from build123d import *

# Parameters (mm, degrees)
F0_R        = 2.4
F1_DEPTH    = 7.88
F2_T1_DEPTH = 26.405


# Not quite as in the source:
# - a fillet or chamfer that OpenCascade refuses, or shapes differently, is made with other operations: its cross-section is extruded or revolved along the edge and cut away or added


with BuildPart() as f1:
    # F0 (on Top) → F1 (new body)
    with BuildSketch(Plane.XY):
        Polygon((-48.3995083171, -5.7841986276), (-31.3221290569, -5.7841986276), (-9.0295083171, -5.7841986276), (-9.0295083171, 1.2940158032), (-41.0095083171, 1.2940158032), (-41.0095083171, 17.5958013724), (-48.3995083171, 17.5958013724), align=None)
        with Locations((-44.7195083171, -2.0891986276)):
            Circle(F0_R, mode=Mode.SUBTRACT)
        with Locations((-36.7195083171, -2.0891986276)):
            Circle(F0_R, mode=Mode.SUBTRACT)
        with BuildLine():
            ThreePointArc((-28.7195083171, -4.4891986276), (-31.1195083171, -2.0891986276), (-28.7195083171, 0.3108013724))
            ThreePointArc((-28.7195083171, 0.3108013724), (-26.3195083171, -2.0891986276), (-28.7195083171, -4.4891986276))
        make_face(mode=Mode.SUBTRACT)
        with BuildLine():
            ThreePointArc((-20.7195083171, -4.4891986276), (-23.1195083171, -2.0891986276), (-20.7195083171, 0.3108013724))
            ThreePointArc((-20.7195083171, 0.3108013724), (-18.3195083171, -2.0891986276), (-20.7195083171, -4.4891986276))
        make_face(mode=Mode.SUBTRACT)
        with BuildLine():
            ThreePointArc((-12.7195083171, -4.4891986276), (-15.1195083171, -2.0891986276), (-12.7195083171, 0.3108013724))
            ThreePointArc((-12.7195083171, 0.3108013724), (-10.3195083171, -2.0891986276), (-12.7195083171, -4.4891986276))
        make_face(mode=Mode.SUBTRACT)
        with Locations((-44.7195083171, 5.9108013724)):
            Circle(F0_R, mode=Mode.SUBTRACT)
        with Locations((-44.7195083171, 13.9108013724)):
            Circle(F0_R, mode=Mode.SUBTRACT)
    extrude(amount=F1_DEPTH)

    # F2: fillet of radius 3.705 on 5 edges, made by hand

    # F2_s2 → F2_t1 (cut)
    with BuildSketch(Plane.XY.offset(-9.2625)):
        with BuildLine():
            ThreePointArc((-48.3995083171, 13.8908013724), (-47.3143389413, 16.5106319967), (-44.6945083171, 17.5958013724))
            Line((-44.6945083171, 17.5958013724), (-48.3995083171, 17.5958013724))
            Line((-48.3995083171, 17.5958013724), (-48.3995083171, 13.8908013724))
        make_face()
        with BuildLine():
            ThreePointArc((-41.0095083171, 13.8908013724), (-42.0946776928, 16.5106319967), (-44.7145083171, 17.5958013724))
            Line((-44.7145083171, 17.5958013724), (-41.0095083171, 17.5958013724))
            Line((-41.0095083171, 17.5958013724), (-41.0095083171, 13.8908013724))
        make_face()
        with BuildLine():
            ThreePointArc((-9.0295083171, -2.4109841968), (-10.1146776928, 0.2088464274), (-12.7345083171, 1.2940158032))
            Line((-12.7345083171, 1.2940158032), (-9.0295083171, 1.2940158032))
            Line((-9.0295083171, 1.2940158032), (-9.0295083171, -2.4109841968))
        make_face()
        with BuildLine():
            ThreePointArc((-9.0295083171, -2.0791986276), (-10.1146776928, -4.6990292519), (-12.7345083171, -5.7841986276))
            Line((-12.7345083171, -5.7841986276), (-9.0295083171, -5.7841986276))
            Line((-9.0295083171, -5.7841986276), (-9.0295083171, -2.0791986276))
        make_face()
        with BuildLine():
            ThreePointArc((-44.6945083171, -5.7841986276), (-47.3143389413, -4.6990292519), (-48.3995083171, -2.0791986276))
            Line((-48.3995083171, -2.0791986276), (-48.3995083171, -5.7841986276))
            Line((-48.3995083171, -5.7841986276), (-44.6945083171, -5.7841986276))
        make_face()
    extrude(amount=F2_T1_DEPTH, mode=Mode.SUBTRACT)


solid = f1.part
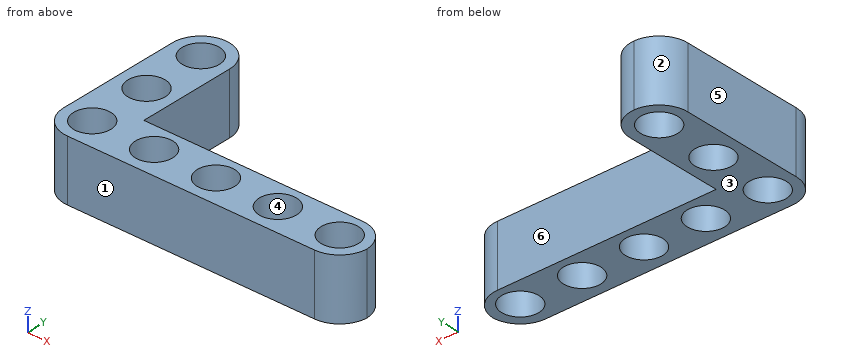
The listing builds one solid part. Answer for the finished solid, in the listing's coordinates (mm). Face numbers are marked on the shaded views. A direction names the side the tool comes from. Coordinates: 2 decimals unless noted, no trailing zeros. Write each loop counter-clockwise with the first axis right and the second up, starting at its lowest first coordinate (ties: lowest second). Pieces come first, ordered by that corner, then holes. Notation, with made-up numbers: (64.5, 36) - (95.5, 36) arc R23 cw to (95.5, 62) - close; hole circle Ø4 at (18, 24.5). An arc over 180 degrees is marked (long way). Return JSON: item names as keys, results as strings.
1. The part is cut by section B-B on z = 5.5. Determine the outline of the cut face in (x, y) (1 decimal).
Final values:
{"outline": "(-48.4, -2.1) arc R3.7 ccw to (-44.7, -5.8) - (-12.7, -5.8) arc R3.7 ccw to (-9, -2.2) arc R3.7 ccw to (-12.7, 1.3) - (-41, 1.3) - (-41, 13.9) arc R3.7 ccw to (-44.7, 17.6) arc R3.7 ccw to (-48.4, 13.9) - close; hole circle Ø4.8 at (-44.7, -2.1); hole circle Ø4.8 at (-44.7, 5.9); hole circle Ø4.8 at (-44.7, 13.9); hole circle Ø4.8 at (-36.7, -2.1); hole circle Ø4.8 at (-28.7, -2.1); hole circle Ø4.8 at (-20.7, -2.1); hole circle Ø4.8 at (-12.7, -2.1)"}
2. Each of these flat-tipped pins is pushed along its axis until it touches: pin 1 Ø4 at (x, y) = (-44.72, 13.91) entering from -Z; pin 2 Ø4 at (y, z) = (0.5, 1.5) entering from +X. Where does it stop, or does it pass through?
Final values:
{"pin 1": "through", "pin 2": "x = -9.14"}
3. The part is cut by section A-A on y = 5. Determine the outline of the cut face in (x, z).
Final values:
{"outline": "(-48.4, 0) - (-46.94, 0) - (-46.94, 7.88) - (-48.4, 7.88) - close; (-42.5, 0) - (-41.01, 0) - (-41.01, 7.88) - (-42.5, 7.88) - close"}
4. For a pull along Y with two mould halves and no side action, classify the marked faces 1, 2, 3 and 4 as +Y half, -Y half, draft (parallel to the pull), parting line (faces both ways), or undercut.
Final values:
{"face 1": "-Y half", "face 2": "+Y half", "face 3": "draft", "face 4": "undercut"}
5. The part is cut by section D-D on x = -25.5. Determine the outline of the cut face in (y, z).
Final values:
{"outline": "(-5.78, 0) - (1.29, 0) - (1.29, 7.88) - (-5.78, 7.88) - close"}
6. The part is cut by section C-C on x = -13.5. Determine the outline of the cut face in (y, z), then the cut area to 3 significant figures.
Final values:
{"outline": "(-5.78, 0) - (-4.36, 0) - (-4.36, 7.88) - (-5.78, 7.88) - close; (0.18, 0) - (1.29, 0) - (1.29, 7.88) - (0.18, 7.88) - close", "area": "20.0 mm^2"}
7. Consider line 1 along X through (y, z) = (5.75, 3.75); line 2 along Y through (x, z) = (-20.5, 5); line 3 along X through (y, z) = (2, 7). Determine where each line is inside the solid, lowest interval first.
Final values:
{"line 1": "-48.4 to -47.11, -42.32 to -41.01", "line 2": "-5.78 to -4.48, 0.3 to 1.29", "line 3": "-48.4 to -41.01"}
8. Which of the six approach directions +Z, -Z, +X, -X, +Y, -Y give full straight-line access (tool end or side, diameter ignored) to the marked faces 5 and 6?
Final values:
{"face 5": "+Z, -Z, -X, +Y, -Y", "face 6": "+Z, -Z, +X, +Y"}
